Design review of the part built by this model. Coordinates are the model's own, in mm. Face numbers are marked on the shaded views. Coordinates: 2 decimals unless noted, no trailing zeros. Write each loop counter-clockwise with the first axis right and the second up, starting at its lowest first coordinate (ties: lowest second). Pieces come first, ordered by that corner, then holes.
Q1. Add section D-D, the plane x = 1.75. Give the boundary of the cut face in (y, z).
Q2. The part is to be moulded in two halves that separate along Y. For the marked faces 1, 2 and 3, say which applies: +Y half, -Y half, draft (parallel to the pull), parting line (faces both ways), or undercut.
Q3. To check wall thickness, follow probe 1 along Y at (x, z) = (12.5, 5); probe 2 along X at (y, z) = (30.5, 4.5); probe 3 along Y at (x, z) = (6.5, 5). State the ranges of each line that lie inside material, in increasing order.
Q4. Clearance check with flat-ended pins moving along their axes: pin 1 Ø12 at (x, y) = (7.5, 31.5) entering from -Z; pin 2 Ø10 at (x, y) = (10.22, 27.88) entering from -Z. State where each tip first meets the part, or that it passes through.
Q5. Add section C-C, the plane x = 13. Give the boundary of the cut face in (y, z).
Q6. Add section B-B, the plane y = 27.88. Give the boundary of the cut face in (x, z).
Q7. Add section A-A, the plane z = 3.5. Give the boundary of the cut face in (x, y) (1 decimal).
from build123d import *

# Parameters (mm, degrees)
SKETCH1_R           = 6.3
BOSS_EXTRUDE1_DEPTH = 9
SKETCH2_R           = 1.505
CUT_EXTRUDE1_DEPTH  = 9


with BuildPart() as part:
    # Sketch1 → Boss-Extrude1 (new body)
    with BuildSketch(Plane.XY):
        with BuildLine():
            Line((0, 0), (20.437665022, 0))
            Line((20.437665022, 0), (24.603832511, 4.166167489))
            Line((24.603832511, 4.166167489), (24.603832511, 33.652501624))
            ThreePointArc((24.603832511, 33.652501624), (10.218832511, 43.38), (-4.166167489, 33.652501624))
            Line((-4.166167489, 33.652501624), (-4.166167489, 4.166167489))
            Line((-4.166167489, 4.166167489), (0, 0))
        make_face()
        with Locations((10.218832511, 27.88)):
            Circle(SKETCH1_R, mode=Mode.SUBTRACT)
    extrude(amount=BOSS_EXTRUDE1_DEPTH)

    # Sketch2 → Cut-Extrude1 (cut)
    with BuildSketch(Plane.XY.offset(9)):
        with Locations((0.718832511, 27.88)):
            Circle(SKETCH2_R)
        with Locations((19.718832511, 27.88)):
            Circle(SKETCH2_R)
    extrude(amount=-CUT_EXTRUDE1_DEPTH, mode=Mode.SUBTRACT)


solid = part.part
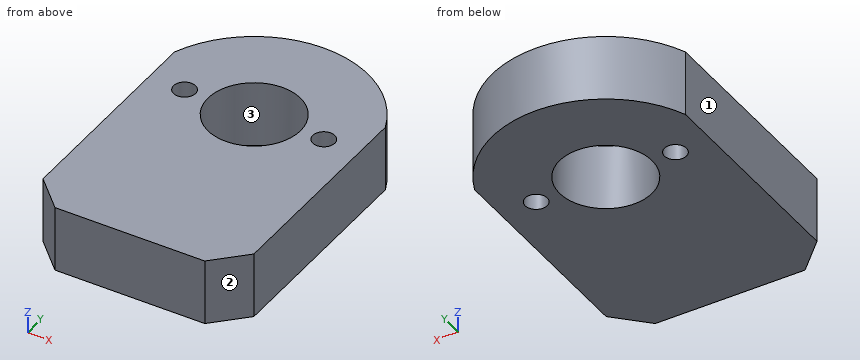
Here are the results:
1. outline: (0, 0) - (26.78, 0) - (26.78, 9) - (0, 9) - close; (28.98, 0) - (40.86, 0) - (40.86, 9) - (28.98, 9) - close
2. face 1: draft
2. face 2: -Y half
2. face 3: undercut
3. probe 1: y = 0 to 22.01, 33.75 to 43.21
3. probe 2: x = -4.17 to 4.49, 15.95 to 24.6
3. probe 3: y = 0 to 22.79, 32.97 to 42.93
4. pin 1: stops at z = 0
4. pin 2: passes through
5. outline: (0, 0) - (22.23, 0) - (22.23, 9) - (0, 9) - close; (33.53, 0) - (43.13, 0) - (43.13, 9) - (33.53, 9) - close
6. outline: (-4.17, 0) - (-0.79, 0) - (-0.79, 9) - (-4.17, 9) - close; (2.22, 0) - (3.92, 0) - (3.92, 9) - (2.22, 9) - close; (16.52, 0) - (18.21, 0) - (18.21, 9) - (16.52, 9) - close; (21.22, 0) - (24.6, 0) - (24.6, 9) - (21.22, 9) - close
7. outline: (-4.2, 4.2) - (0, 0) - (20.4, 0) - (24.6, 4.2) - (24.6, 33.7) arc R15.5 ccw to (-4.2, 33.7) - close; hole circle Ø3 at (0.7, 27.9); hole circle Ø12.6 at (10.2, 27.9); hole circle Ø3 at (19.7, 27.9)
